Drawing for the job (mm, zero at the part's lowest x, y, z). Give positions to 0.01 mm unless a question says otherwise; leave off trailing zeros. Write each loop counter-clockwise with the first axis right and the second up, starting at its lowest first coordinate (ties: lowest second). Pieces come first, ordered by that corner, then holes. Notation, with made-up numbers: M 8.5,84 L 51.5,84 A19 cw 51.5,98 Z; hole C 1.25,54 d6. An arc over 180 degrees is marked long. Use CSV: the item, a comma, the result in double quotes. Start each with the question number.
1. Band-saw the part on B-B, the plane y = 0.9. List the corners of the cut face in (x, z), then the cut area to 3 significant figures.
2. Band-saw the part on A-A, the plane z = 45. List the corners of the cut face in (x, y).
3. Drill centre line: line 1 along X through (y, z) = (0.2, 16.5). Where is it in solid material? Low to high. Write a range as from..to.
4. Mould opens along Y. For the marked faces 1 and 2 say: pulls with the +Y half, pulls with the -Y half, needs draft (parallel to the pull), parting line crosses it, or undercut.
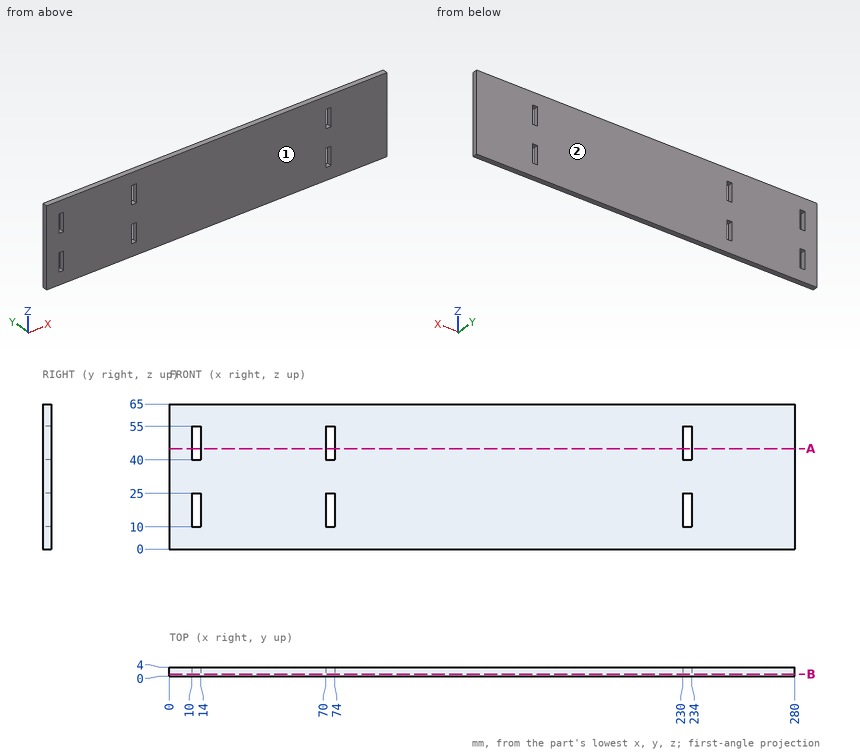
Output:
1,outline,"M 0,0 L 280,0 L 280,65 L 0,65 Z; hole M 10,10 L 14,10 L 14,25 L 10,25 Z; hole M 10,40 L 14,40 L 14,55 L 10,55 Z; hole M 70,10 L 74,10 L 74,25 L 70,25 Z; hole M 70,40 L 74,40 L 74,55 L 70,55 Z; hole M 230,10 L 234,10 L 234,25 L 230,25 Z; hole M 230,40 L 234,40 L 234,55 L 230,55 Z"
1,area,"17,800 mm²"
2,outline,"M 0,0 L 10,0 L 10,4 L 0,4 Z; M 14,0 L 70,0 L 70,4 L 14,4 Z; M 74,0 L 230,0 L 230,4 L 74,4 Z; M 234,0 L 280,0 L 280,4 L 234,4 Z"
3,line 1,"x = 0..10, 14..70, 74..230, 234..280"
4,face 1,"pulls with the -Y half"
4,face 2,"pulls with the +Y half"
